Could you check a few things on this drawing? It's one solid part, dimensions in mm from its lowest x, y, z. A direction names the side the tool comes from. Give positions to 0.01 mm unless a question says otherwise; leave off trailing zeros. Loops run counter-clockwise (first coordinate to the right, second up) from the corner with the lowest first, then second, coordinate; pieces in that order, holes last.
Q1. Suppose I cut it at B-B (z = 11.5). List the corners of the cut face in (x, y) for me, and give its area (3 significant figures).
Q2. I need wall thicknesses on probe 1 along X at (y, z) = (39, 1); probe 2 along X at (y, z) = (26.5, 6.75); probe 3 along Y at (x, z) = (19, 6.75). Which ranges of each line are inside material? Lowest first, please.
Q3. For the marked faces 1, 2 and 3, which set-ups out of +Z, -Z, +X, -X, +Y, -Y let a thin tool reach every point of the face, with its end or its side?
Q4. Suppose I cut it at C-C (y = 40). List the corners of the cut face in (x, z) for me.
Q5. I'm going to push flat-ended pins straight in: P1, Ø12, axis at x = 22, y = 31.5, coming from the -Z side; P2, Ø3, axis at x = 6, z = 5.5, coming from the +Y side; P3, Ø1.5, axis at x = 46, z = 4.5, coming from the -Y side. Where does each tip first touch, or does it pass through?
Q6. Thinking about a two-plate mould opening in X: for the marked faces 4, 5 and 6, which applies, pulls with the +X half, pulls with the -X half, needs draft (parallel to the pull), parting line crosses it, or undercut?
Q7. Suppose I cut it at A-A (y = 47.4). List the corners of the cut face in (x, z) for me.
Q8. Suppose I cut it at D-D (x = 4.5). List the corners of the cut face in (y, z) for me, and give its area (3 significant figures).
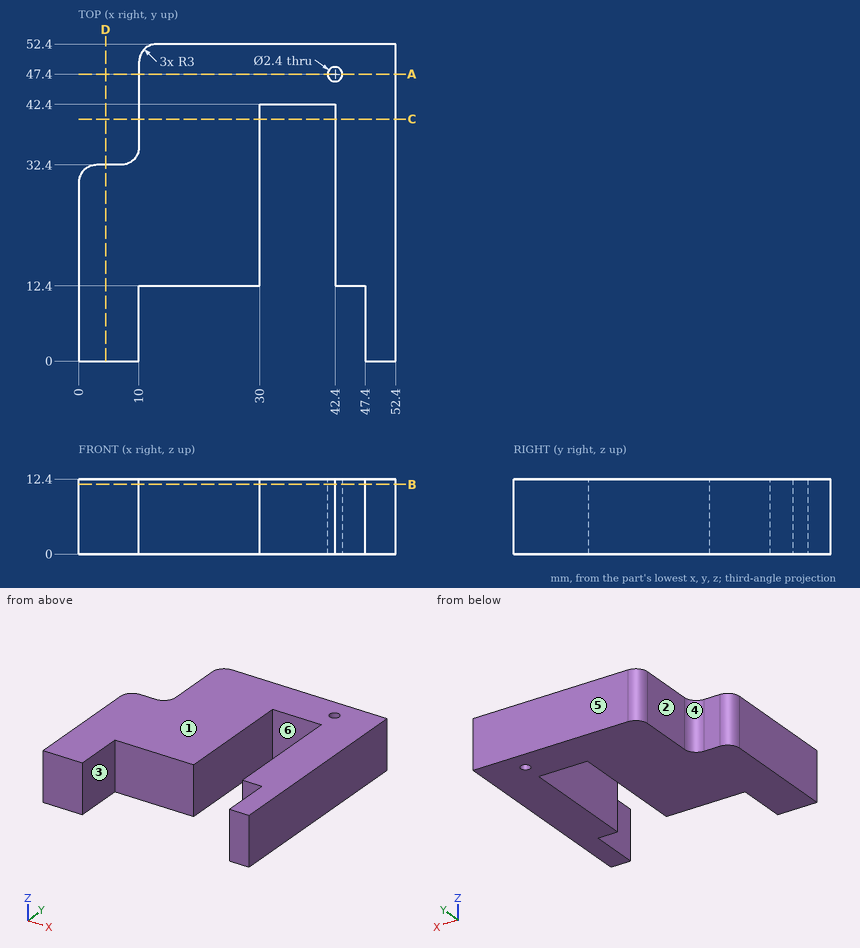
Solutions:
1. outline: (0, 0) - (10, 0) - (10, 12.4) - (30, 12.4) - (30, 42.4) - (42.4, 42.4) - (42.4, 12.4) - (47.4, 12.4) - (47.4, 0) - (52.4, 0) - (52.4, 52.4) - (13, 52.4) arc R3 ccw to (10, 49.4) - (10, 35.4) arc R3 cw to (7, 32.4) - (3, 32.4) arc R3 ccw to (0, 29.4) - close; hole circle Ø2.4 at (42.4, 47.4)
1. area: 1,700 mm2
2. probe 1: x = 10 to 30, 42.4 to 52.4
2. probe 2: x = 0 to 30, 42.4 to 52.4
2. probe 3: y = 12.4 to 52.4
3. face 1: +Z, +X, -X, +Y, -Y
3. face 2: +Z, -Z, -X, +Y
3. face 3: +Z, -Z, -Y
4. outline: (10, 0) - (30, 0) - (30, 12.4) - (10, 12.4) - close; (42.4, 0) - (52.4, 0) - (52.4, 12.4) - (42.4, 12.4) - close
5. P1: stops at z = 0
5. P2: stops at y = 32.44
5. P3: stops at y = 12.4
6. face 4: pulls with the -X half
6. face 5: needs draft
6. face 6: undercut
7. outline: (10, 0) - (41.2, 0) - (41.2, 12.4) - (10, 12.4) - close; (43.6, 0) - (52.4, 0) - (52.4, 12.4) - (43.6, 12.4) - close
8. outline: (0, 0) - (32.4, 0) - (32.4, 12.4) - (0, 12.4) - close
8. area: 402 mm2
